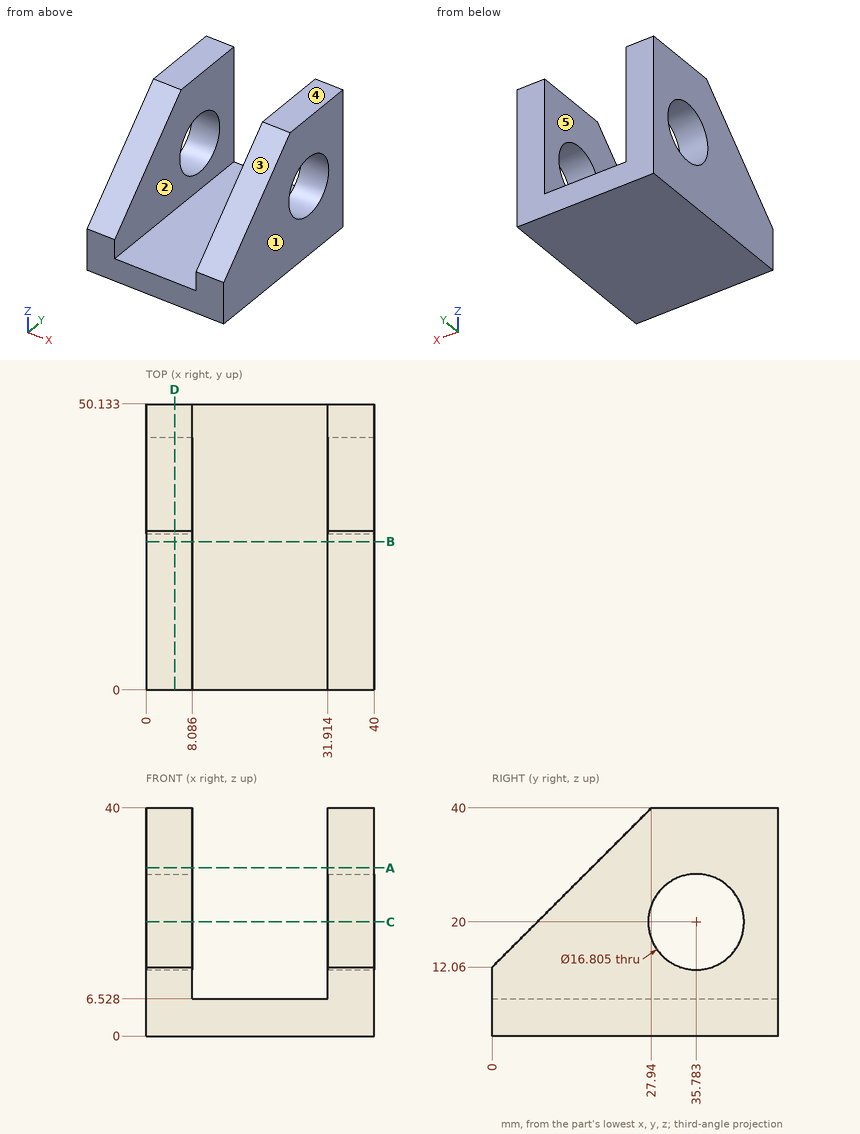
Verification items for this drawing (mm, ordinates from the low corner). A direction names the side the tool comes from. Give positions to 0.01 mm unless a question says otherwise; leave off trailing zeros. Loops run counter-clockwise (first coordinate to the right, second up) from the corner with the lowest first, then second, coordinate; pieces in that order, holes last. Notation, with made-up numbers: (46.25, -17) - (55.25, -17) arc R9 cw to (55.25, 0) - close; hole circle Ø5 at (86, 76). An arc over 180 degrees is marked (long way). Write item = value, one per line. Start each with the question number.
Q1. Thickness scan on line 1 (X direction, y = 15.5, z = 26) (1 decimal); line 2 (Z direction, x = 17.5, y = 3.5); line 3 (Z direction, x = 3, y = 37). Record the ranges inside material, lowest first.
Q2. Cross-section at C-C, the plane z = 20. Enter the section's corners in (x, y) (1 decimal).
Q3. Mould release check, pull along X, two halves, no side actions. Record for the marked faces 1, 2 and 3: released by +X, released by -X, zero draft, split by the parting line, or undercut.
Q4. Cross-section at D-D, the plane x = 5. Enter the section's corners in (y, z) (1 decimal), and give its area (3 significant figures).
Q5. Cross-section at B-B, the plane y = 26. Enter the section's corners in (x, z) (1 decimal).
Q6. Depth check by flat-ended pin: P1, Ø8, axis at x = 24.5, y = 28.5, coming from the +Z side; P2, Ø15, axis at y = 35.78, z = 20, coming from the -X side; P3, Ø3, axis at x = 35.5, y = 14.5, coming from the +Z side. Enter the tip coordinate at first touch or a pass-through.
Q7. Cross-section at A-A, the plane z = 29.5. Enter the section's corners in (x, y) (1 decimal), and give its area (3 significant figures).
Q8. Tool access check on the marked faces 4 and 5. Record the directions out of +Z, -Z, +X, -X, +Y, -Y that give a thin tool (end or side, any length) a straight path to the whole face; none if there is none.
Answer key:
q1.line_1 = 0 to 8.1, 31.9 to 40
q1.line_2 = 0 to 6.53
q1.line_3 = 0 to 11.69, 28.31 to 40
q2.outline = (0, 7.9) - (8.1, 7.9) - (8.1, 27.4) - (0, 27.4) - close; (0, 44.2) - (8.1, 44.2) - (8.1, 50.1) - (0, 50.1) - close; (31.9, 7.9) - (40, 7.9) - (40, 27.4) - (31.9, 27.4) - close; (31.9, 44.2) - (40, 44.2) - (40, 50.1) - (31.9, 50.1) - close
q3.face_1 = released by +X
q3.face_2 = undercut
q3.face_3 = zero draft
q4.outline = (0, 0) - (50.1, 0) - (50.1, 40) - (27.9, 40) - (0, 12.1) - close; hole circle Ø16.8 at (35.8, 20)
q4.area = 1,390 mm^2
q5.outline = (0, 0) - (40, 0) - (40, 38.1) - (31.9, 38.1) - (31.9, 6.5) - (8.1, 6.5) - (8.1, 38.1) - (0, 38.1) - close
q6.P1 = 6.53
q6.P2 = through
q6.P3 = 28.06
q7.outline = (0, 17.4) - (8.1, 17.4) - (8.1, 50.1) - (0, 50.1) - close; (31.9, 17.4) - (40, 17.4) - (40, 50.1) - (31.9, 50.1) - close
q7.area = 529 mm^2
q8.face_4 = +Z, +X, -X, +Y, -Y
q8.face_5 = +Z, +Y, -Y
